```python
from build123d import *

# Parameters (mm, degrees)
SKETCH1_R           = 4
BOSS_EXTRUDE1_DEPTH = 10


with BuildPart() as part:
    # Sketch1 → Boss-Extrude1 (new body)
    with BuildSketch(Plane.XY):
        with BuildLine():
            Line((24.494897428, 149.96344327), (-90, 149.96344327))
            Line((-90, 149.96344327), (-115, 122.96344327))
            Line((-115, 122.96344327), (-101.371578153, 122.96344327))
            Line((-101.371578153, 122.96344327), (-85.630837413, 139.96344327))
            Line((-85.630837413, 139.96344327), (-24.494897428, 139.96344327))
            ThreePointArc((-24.494897428, 139.96344327), (-24.117560965, 138.379883968), (-23.63796439, 136.824239409))
            ThreePointArc((-23.63796439, 136.824239409), (-22.00386591, 136.155983342), (-20.251106776, 136.367358443))
            Line((-20.251106776, 136.367358443), (-17.029339789, 137.734917393))
            ThreePointArc((-17.029339789, 137.734917393), (-16.02146997, 135.71344327), (-14.774756936, 133.829865342))
            Line((-14.774756936, 133.829865342), (-17.569981221, 131.723512761))
            ThreePointArc((-17.569981221, 131.723512761), (-18.629416995, 130.311266375), (-18.867739506, 128.561967545))
            ThreePointArc((-18.867739506, 128.561967545), (-17.67766953, 127.28577374), (-16.401475725, 126.095703764))
            ThreePointArc((-16.401475725, 126.095703764), (-14.652176895, 126.334026275), (-13.239930509, 127.393462049))
            Line((-13.239930509, 127.393462049), (-11.133577928, 130.188686334))
            ThreePointArc((-11.133577928, 130.188686334), (-9.25, 128.9419733), (-7.228525877, 127.934103481))
            Line((-7.228525877, 127.934103481), (-8.596084827, 124.712336494))
            ThreePointArc((-8.596084827, 124.712336494), (-8.807459928, 122.95957736), (-8.139203861, 121.32547888))
            ThreePointArc((-8.139203861, 121.32547888), (-6.470476128, 120.815297613), (-4.770224884, 120.422763684))
            ThreePointArc((-4.770224884, 120.422763684), (-3.374448914, 121.503806447), (-2.681125555, 123.127427934))
            Line((-2.681125555, 123.127427934), (-2.254582853, 126.601339465))
            ThreePointArc((-2.254582853, 126.601339465), (0, 126.46344327), (2.254582853, 126.601339465))
            Line((2.254582853, 126.601339465), (2.681125555, 123.127427934))
            ThreePointArc((2.681125555, 123.127427934), (3.374448914, 121.503806447), (4.770224884, 120.422763684))
            ThreePointArc((4.770224884, 120.422763684), (6.470476128, 120.815297613), (8.139203861, 121.32547888))
            ThreePointArc((8.139203861, 121.32547888), (8.807459928, 122.95957736), (8.596084827, 124.712336494))
            Line((8.596084827, 124.712336494), (7.228525877, 127.934103481))
            ThreePointArc((7.228525877, 127.934103481), (9.25, 128.9419733), (11.133577928, 130.188686334))
            Line((11.133577928, 130.188686334), (13.239930509, 127.393462049))
            ThreePointArc((13.239930509, 127.393462049), (14.652176895, 126.334026275), (16.401475725, 126.095703764))
            ThreePointArc((16.401475725, 126.095703764), (17.67766953, 127.28577374), (18.867739506, 128.561967545))
            ThreePointArc((18.867739506, 128.561967545), (18.629416995, 130.311266375), (17.569981221, 131.723512761))
            Line((17.569981221, 131.723512761), (14.774756936, 133.829865342))
            ThreePointArc((14.774756936, 133.829865342), (16.02146997, 135.71344327), (17.029339789, 137.734917393))
            Line((17.029339789, 137.734917393), (20.251106776, 136.367358443))
            ThreePointArc((20.251106776, 136.367358443), (22.00386591, 136.155983342), (23.63796439, 136.824239409))
            ThreePointArc((23.63796439, 136.824239409), (24.148145657, 138.492967142), (24.540679586, 140.193218386))
            ThreePointArc((24.540679586, 140.193218386), (23.459636823, 141.588994356), (21.836015336, 142.282317715))
            Line((21.836015336, 142.282317715), (18.362103805, 142.708860417))
            ThreePointArc((18.362103805, 142.708860417), (18.5, 144.96344327), (18.362103805, 147.218026123))
            Line((18.362103805, 147.218026123), (21.836015336, 147.644568825))
            ThreePointArc((21.836015336, 147.644568825), (23.459636823, 148.337892184), (24.540679586, 149.733668154))
            ThreePointArc((24.540679586, 149.733668154), (24.518057681, 149.848609344), (24.494897428, 149.96344327))
        make_face()
        with Locations((0, 144.96344327)):
            Circle(SKETCH1_R, mode=Mode.SUBTRACT)
    extrude(amount=BOSS_EXTRUDE1_DEPTH)


solid = part.part
```
Here's how the part is built. I have some questions about the finished solid (model axes, mm). A direction names the side the tool comes from. Give positions to 0.01 mm unless a question says otherwise; leave off trailing zeros. Loops run counter-clockwise (first coordinate to the right, second up) from the corner with the lowest first, then second, coordinate; pieces in that order, holes last. Notation, with made-up numbers: M -27,78 L -22,78 A23 cw -22,109 Z; hole C 79,12.25 d8. An arc over 180 degrees is marked long. Put each result on its own line as item: value. Start each with the question number.
(1) I want a section at B-B on x = -83.5. Please give me the cut outline in (y, z).
(2) If we mould it in two halves opening along X, with no side actions, what happens to faces 4 (the cylindrical face through (23.44, 148.323, 4.93)), 5 (the flat face through (-2.47, 124.84, 4.93)), 6 (the flat face through (-31, 142, 0)), 7 (the cylindrical face through (16.01, 135.69, 4.93))? For each: +X half, -X half, draft (parallel to the pull), parting line (faces both ways), or undercut.
(3) For faces 1 (the cylindrical face through (-8.81, 122.98, 4.93)), 2 (the flat face through (20.075, 147.428, 4.93)), 3 (the cylindrical face through (3.36, 121.52, 4.93)), which set-ups out of +Z, -Z, +X, -X, +Y, -Y let a thin tool reach every point of the face, with its end or its side?
(4) Will these pins go through, and if not, where does the flat tip stop? pin 1 Ø5 at (x, z) = (-32.5, 4.5) entering from -Y; pin 2 Ø7 at (x, y) = (0, 144.96) entering from +Z; pin 3 Ø4 at (y, z) = (126.5, 8.5) entering from +X; pin 4 Ø2 at (y, z) = (130, 6) entering from +X.
(5) I want a section at A-A on x = 0. Please give me the cut outline in (y, z).
(6) I need wall thicknesses on line 1 along Y through (x, z) = (0, 4.75); line 2 along X through (y, z) = (128.75, 5.25); line 3 along X through (y, z) = (125, 8.5). Which ranges of each line are inside material? Lowest first, please. Write a range as [from, to].
Answer block:
1. outline: M 139.96,0 L 149.96,0 L 149.96,10 L 139.96,10 Z
2. face 4: +X half
2. face 5: undercut
2. face 6: draft
2. face 7: undercut
3. face 1: +Z, -Z
3. face 2: +Z, -Z, +X
3. face 3: +Z, -Z, -Y
4. pin 1: y = 139.96
4. pin 2: through
4. pin 3: x = 18.81
4. pin 4: x = 18.89
5. outline: M 126.46,0 L 140.96,0 L 140.96,10 L 126.46,10 Z; M 148.96,0 L 149.96,0 L 149.96,10 L 148.96,10 Z
6. line 1: [126.46, 140.96], [148.96, 149.96]
6. line 2: [-109.64, -96.01], [-18.89, -12.22], [-8.91, 8.91], [12.22, 18.89]
6. line 3: [-113.11, -99.49], [-8.47, -2.45], [2.45, 8.47]
